Source: CAD feature listing. Evaluate the final solid. Frame: model axes, mm. Face numbers are marked on the shaded views. A direction names the side the tool comes from. Coordinates: 2 decimals unless noted, no trailing zeros. Write each loop counter-clockwise with the first axis right and the second up, starting at its lowest first coordinate (ties: lowest second). Pieces come first, ordered by that corner, then holes. Notation, with made-up numbers: (18, 79.25) - (53, 79.25) arc R23 ccw to (53, 114.25) - close; hole circle Ø1 at (38.25, 62.5). An arc over 180 degrees is marked (long way). One line per question, with ' | ' between items. Start each with the question number.
Q1. Cut plane D-D, the plane z = 28.5. Return loops of the section in (x, y), plus the area to 3 significant figures.
Q2. Cut plane C-C, the plane y = -26. Return loops of the section in (x, z), plus the area to 3 significant figures.
Q3. Cut plane B-B, the plane x = -1. Return loops of the section in (y, z).
Q4. Line query: line 1 (X direction, y = -35, z = 12); line 2 (Z direction, x = -15.25, y = -22.5); line 3 (Z direction, x = -4, y = -36). Output: solid intervals per line, ascending.
Q5. Cut plane A-A, the plane y = -19.05. Return loops of the section in (x, z), plus the area to 3 significant figures.
Q6. Access query for the marked faces 1, 2 and 3. Directions: +Z, -Z, +X, -X, +Y, -Y. A direction counts if a zero-diameter tool reaches every point of the face in a straight line with its end or side. Return the directions, or none.
Q7. Contact query for flat-ended pins moving along their axis: P1, Ø1.7, axis at y = -23, z = -1.5, coming from the -X side; P2, Ø8, axis at x = -8.5, z = 32.5, coming from the +Y side; P3, Ø8, axis at x = -11, y = -13, coming from the +Z side; P4, Ø0.9, axis at x = -17, y = -27, coming from the +Z side. Output: stop coordinate, or through.
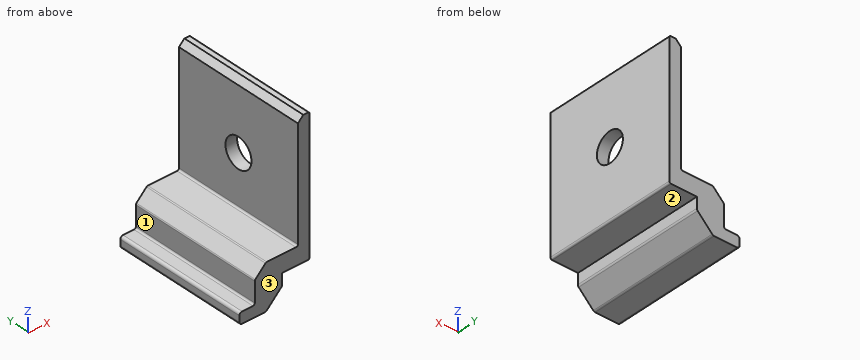
```python
from build123d import *

# Parameters (mm, degrees)
BOSS_EXTRUDE1_DEPTH = 38.1
SKETCH2_W           = 3.175
SKETCH2_H           = 38.1
BOSS_EXTRUDE2_DEPTH = 4.3688
HOLE1_D             = 8.3312
HOLE1_DEPTH         = 19.862825
FILLET1_R           = 0.508
FILLET2_R           = 0.762


with BuildPart() as part:
    # Sketch1 → Boss-Extrude1 (new body)
    with BuildSketch(Plane(origin=(0, 0, 0), x_dir=(1, 0, 0), z_dir=(0, 1, 0))):
        Polygon((-12.236871502, 8.069451482), (-15.386471502, 8.069451482), (-15.386471502, -1.455548518), (-12.211471502, -4.630548518), (-3.194471502, -4.630548518), (-3.194471502, -36.263708518), (-1.670471502, -37.787708518), (0.107528498, -37.787708518), (0.107528498, 0.195451482), (-7.664871502, 0.195451482), (-7.664871502, 3.497451482), align=None)
    extrude(amount=-BOSS_EXTRUDE1_DEPTH)

    # Sketch2 → Boss-Extrude2 (add)
    with BuildSketch(Plane.ZY.offset(15.386471502)):
        with Locations((-6.481951482, -19.05)):
            Rectangle(SKETCH2_W, SKETCH2_H)
    extrude(amount=BOSS_EXTRUDE2_DEPTH)

    # Hole1
    with Locations(Plane(origin=(0.107528498, 0, 0), x_dir=(0, 0, -1), z_dir=(1, 0, 0))):
        with Locations((-18.854548518, -19.05)):
            Hole(HOLE1_D / 2, depth=HOLE1_DEPTH)

    # Fillet1
    fillet1_edges = [part.edges().sort_by_distance(p)[0] for p in [
        (-15.386471502, -19.05, -4.894451482),
        (0.107528498, -19.05, -0.195451482),
        (0.107528498, -19.05, 37.787708518),
        (-12.211471502, -19.05, 4.630548518),
        (-3.194471502, -19.05, 4.630548518),
        (-15.386471502, -19.05, 1.455548518),
    ]]
    fillet(fillet1_edges, radius=FILLET1_R)

    # Fillet2
    fillet2_edges = [part.edges().sort_by_distance(p)[0] for p in [
        (-7.664871502, -19.05, -3.497451482),
        (-19.755271502, -19.05, -4.894451482),
        (-19.755271502, -19.05, -8.069451482),
        (-12.236871502, -19.05, -8.069451482),
    ]]
    fillet(fillet2_edges, radius=FILLET2_R)


solid = part.part
```
Reply:
1) outline: (-3.19, -38.1) - (0.11, -38.1) - (0.11, 0) - (-3.19, 0) - close | area: 126 mm^2
2) outline: (-19.76, -7.31) arc R0.76 ccw to (-18.99, -8.07) - (-12.55, -8.07) arc R0.76 ccw to (-12.01, -7.85) - (-7.89, -3.72) arc R0.76 ccw to (-7.66, -3.18) - (-7.66, -0.2) - (-0.4, -0.2) arc R0.51 ccw to (0.11, 0.31) - (0.11, 37.28) arc R0.51 ccw to (-0.4, 37.79) - (-1.67, 37.79) - (-3.19, 36.26) - (-3.19, 5.14) arc R0.51 cw to (-3.7, 4.63) - (-12, 4.63) arc R0.51 ccw to (-12.36, 4.48) - (-15.24, 1.6) arc R0.51 ccw to (-15.39, 1.25) - (-15.39, -4.39) arc R0.51 cw to (-15.89, -4.89) - (-18.99, -4.89) arc R0.76 ccw to (-19.76, -5.66) - close | area: 242 mm^2
3) outline: (-38.1, -0.2) - (0, -0.2) - (0, 37.79) - (-38.1, 37.79) - close; hole circle Ø8.33 at (-19.05, 18.85)
4) line 1: x = -3.19 to 0.11 | line 2: z = -8.07 to 1.59 | line 3: z = -0.2 to 4.63
5) outline: (-19.76, -7.31) arc R0.76 ccw to (-18.99, -8.07) - (-12.55, -8.07) arc R0.76 ccw to (-12.01, -7.85) - (-7.89, -3.72) arc R0.76 ccw to (-7.66, -3.18) - (-7.66, -0.2) - (-0.4, -0.2) arc R0.51 ccw to (0.11, 0.31) - (0.11, 14.69) - (-3.19, 14.69) - (-3.19, 5.14) arc R0.51 cw to (-3.7, 4.63) - (-12, 4.63) arc R0.51 ccw to (-12.36, 4.48) - (-15.24, 1.6) arc R0.51 ccw to (-15.39, 1.25) - (-15.39, -4.39) arc R0.51 cw to (-15.89, -4.89) - (-18.99, -4.89) arc R0.76 ccw to (-19.76, -5.66) - close; (-3.19, 23.02) - (0.11, 23.02) - (0.11, 37.28) arc R0.51 ccw to (-0.4, 37.79) - (-1.67, 37.79) - (-3.19, 36.26) - close | area: 214 mm^2
6) face 1: +Z, -X, +Y, -Y | face 2: -Z, +X, +Y, -Y | face 3: +Z, -Z, +X, -X, -Y
7) P1: stops at x = -15.39 | P2: passes through | P3: stops at z = 4.63 | P4: stops at z = -4.89
